from build123d import *

# Parameters (mm, degrees)
SKETCH_1_R      = 1.5
SKETCH_1_R_2    = 0.5
EXTRUDE_1_DEPTH = 3


with BuildPart() as part:
    # 草图1 → 凸台-拉伸1 (new body)
    with BuildSketch(Plane(origin=(0, 0, 0), x_dir=(1, 0, 0), z_dir=(0, 1, 0))):
        with BuildLine():
            Line((10, 0), (136.884360712, 0))
            ThreePointArc((136.884360712, 0), (137.900113715, -0.277140216), (138.634360712, -1.031754163))
            Line((138.634360712, -1.031754163), (139.429147615, -2.468245837))
            ThreePointArc((139.429147615, -2.468245837), (140.163394612, -3.222859784), (141.179147615, -3.5))
            Line((141.179147615, -3.5), (168.820852385, -3.5))
            ThreePointArc((168.820852385, -3.5), (169.836605388, -3.222859784), (170.570852385, -2.468245837))
            Line((170.570852385, -2.468245837), (171.365639288, -1.031754163))
            ThreePointArc((171.365639288, -1.031754163), (172.099886285, -0.277140216), (173.115639288, 0))
            Line((173.115639288, 0), (300, 0))
            ThreePointArc((300, 0), (307.071067812, -2.928932188), (310, -10))
            Line((310, -10), (310, -210))
            ThreePointArc((310, -210), (307.071067812, -217.071067812), (300, -220))
            Line((300, -220), (10, -220))
            ThreePointArc((10, -220), (2.928932188, -217.071067812), (0, -210))
            Line((0, -210), (0, -10))
            ThreePointArc((0, -10), (2.928932188, -2.928932188), (10, 0))
        make_face()
        with Locations(Location((14, -14, 0), (0, 0, 270))):
            Circle(SKETCH_1_R, mode=Mode.SUBTRACT)
        with Locations(Location((14, -206, 0), (0, 0, 270))):
            Circle(SKETCH_1_R, mode=Mode.SUBTRACT)
        with Locations(Location((296, -206, 0), (0, 0, 270))):
            Circle(SKETCH_1_R, mode=Mode.SUBTRACT)
        with Locations(Location((296, -12.28568254, 0), (0, 0, 270))):
            Circle(SKETCH_1_R, mode=Mode.SUBTRACT)
        with Locations(Location((155, -206, 0), (0, 0, 270))):
            Circle(SKETCH_1_R, mode=Mode.SUBTRACT)
        with Locations(Location((175, -14, 0), (0, 0, 270))):
            Circle(SKETCH_1_R, mode=Mode.SUBTRACT)
        with Locations(Location((135, -14, 0), (0, 0, 270))):
            Circle(SKETCH_1_R, mode=Mode.SUBTRACT)
        with Locations(Location((296, -110, 0), (0, 0, 270))):
            Circle(SKETCH_1_R, mode=Mode.SUBTRACT)
        with Locations(Location((14, -110, 0), (0, 0, 270))):
            Circle(SKETCH_1_R, mode=Mode.SUBTRACT)
        with Locations(Location((152, -16, 0), (0, 0, 270))):
            Circle(SKETCH_1_R_2, mode=Mode.SUBTRACT)
        Polygon((184.455213096, -18.25), (188.75, -14.75), (285, -14.75), (285, -195), (25, -195), (25, -14.75), (119.25, -14.75), (123.544786904, -18.25), (141.179147615, -18.25), (168.820852385, -18.25), align=None, mode=Mode.SUBTRACT)
    extrude(amount=EXTRUDE_1_DEPTH)


solid = part.part
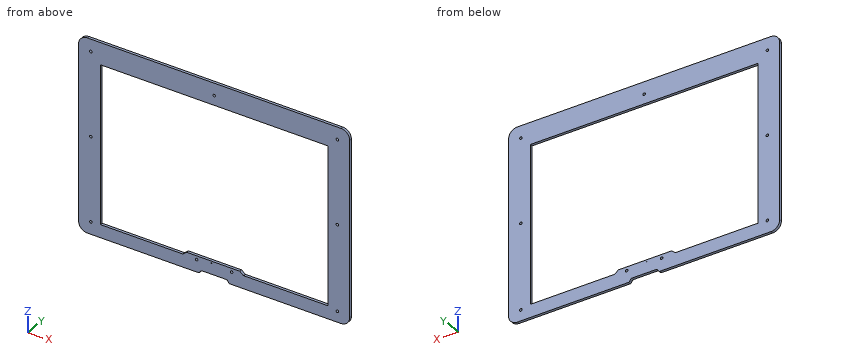
Here's how the part is built. I have some questions about the finished solid (model axes, mm). Give positions to 0.01 mm unless a question says otherwise; leave off trailing zeros. Order: outer loops, then holes, each group sorted by start corner. A loop starts at its lowest first (then second) coordinate and runs counter-clockwise, first axis right, second up. Notation, with made-up numbers: M -21.5,28.5 L 33.5,28.5 A19 ccw 33.5,41.5 Z; hole C 46,69 d1. An arc over 180 degrees is marked long. Answer as a JSON object with one key per item and string values. Group by question number.
1) Suppose I cut it at B-B, the plane z = 120.5. Write out the boundary of the cut face in (x, y).
2) Suppose I cut it at A-A, the plane x = 253. Write out the boundary of the cut face in (y, z), plus the area to 3 significant figures.
3) Please list where these lines run through material, in increasing order: L1, parallel to Z at x = 175, y = 1.9; L2, parallel to X at y = 0.7, z = 110; L3, parallel to X at y = 1.1, z = 14. Write a range as [from, to].
4) Suppose I cut it at C-C, the plane y = 1.9. Count the separate pieces of the cut face and the enclosed holes in it, plus the area to 3 significant figures.
Results found:
{
 "1": {"outline": "M 0,0 L 25,0 L 25,3 L 0,3 Z; M 285,0 L 310,0 L 310,3 L 285,3 Z"},
 "2": {"outline": "M 0,0 L 3,0 L 3,14.75 L 0,14.75 Z; M 0,195 L 3,195 L 3,220 L 0,220 Z", "area": "119 mm²"},
 "3": {"L1": "[0, 12.5], [15.5, 18.25], [195, 220]", "L2": "[0, 12.5], [15.5, 25], [285, 294.5], [297.5, 310]", "L3": "[0, 12.5], [15.5, 133.5], [136.5, 173.5], [176.5, 310]"},
 "4": {"separate pieces": "1", "enclosed holes": "11", "area": "21,300 mm²"}
}
